Design review of the part built by this model. Coordinates are the model's own, in mm. A direction names the side the tool comes from. Round coordinates to 2 decimals unless told otherwise and drop trailing zeros. Write each loop counter-clockwise with the first axis right and the second up, starting at its lowest first coordinate (ties: lowest second). Pieces come first, ordered by that corner, then holes. Notation, with made-up numbers: M 48.5,55.25 L 101.5,55.25 A11 ccw 101.5,67.25 Z; hole C -34.75,-25 d8. An arc over 180 degrees is marked long. Use CSV: the item, a comma, the result in double quotes.
from build123d import *

# Parameters (mm, degrees)
SKETCH1_W           = 50
SKETCH1_H           = 35
BOSS_EXTRUDE1_DEPTH = 3
SKETCH3_W           = 50
SKETCH3_H           = 3
BOSS_EXTRUDE2_DEPTH = 25
FILLET1_R           = 2
FILLET2_R           = 2


with BuildPart() as part:
    # Sketch1 → Boss-Extrude1 (new body)
    with BuildSketch(Plane.XY):
        Rectangle(SKETCH1_W, SKETCH1_H)
    extrude(amount=BOSS_EXTRUDE1_DEPTH)

    # Sketch3 → Boss-Extrude2 (add)
    with BuildSketch(Plane.XY.offset(3)):
        with Locations((0, -16)):
            Rectangle(SKETCH3_W, SKETCH3_H)
    extrude(amount=BOSS_EXTRUDE2_DEPTH)

    # Fillet1
    fillet1_edges = [part.edges().sort_by_distance(p)[0] for p in [
        (0, -14.5, 3),
    ]]
    fillet(fillet1_edges, radius=FILLET1_R)

    # Fillet2
    fillet2_edges = [part.edges().sort_by_distance(p)[0] for p in [
        (-25, -16, 28),
        (25, -16, 28),
        (-25, 17.5, 1.5),
        (25, 17.5, 1.5),
    ]]
    fillet(fillet2_edges, radius=FILLET2_R)


solid = part.part
1) Add section B-B on y = 13.5. Write out the cut boundary in (x, z).
Answers:
outline,"M -25,0 L 25,0 L 25,3 L -25,3 Z"
2) For pin 1 Ø12 at (y, z) = (10.5, 12) entering from +X; pin 2 Ø4 at (x, y) = (-10, 11.5) entering from +Z; pin 3 Ø4 at (x, z) = (12.5, 21) entering from +Y, all flat-tipped, find the tip position at first contact; note any pin that passes through.
Answers:
pin 1,"through"
pin 2,"z = 3"
pin 3,"y = -14.5"
3) Wall thickness on line 1 along Z through (x, y) = (-11, 10.5); line 2 along Y through (x, z) = (-16.5, 21); line 3 along Y through (x, z) = (-8.5, 3.25): over which ranges is each line inside the solid? List them lowest first. Write a range as [from, to].
Answers:
line 1,"[0, 3]"
line 2,"[-17.5, -14.5]"
line 3,"[-17.5, -13.47]"
4) Add section A-A on x = -10.5. Write out the cut boundary in (y, z).
Answers:
outline,"M -17.5,0 L 17.5,0 L 17.5,3 L -12.5,3 A2 cw -14.5,5 L -14.5,28 L -17.5,28 Z"
5) Add section C-C on z = 6.5. Write out the cut boundary in (x, y).
Answers:
outline,"M -25,-17.5 L 25,-17.5 L 25,-14.5 L -25,-14.5 Z"
6) Machinability: for faces 1 (the face through (-24.43, 16.9, 1.52)), 2 (the face through (0, -14.5, 16)), which of the approach directions +Z, -Z, +X, -X, +Y, -Y give a long, thin tool a straight path to every point of the face, cutting with its end or side? Answer none if there is none.
Answers:
face 1,"+Z, -Z, -X, +Y"
face 2,"+Z, +X, -X, +Y"
